Part model, mm, in its own coordinate system. A direction names the side the tool comes from. Round coordinates to 2 decimals unless told otherwise and drop trailing zeros. Loops run counter-clockwise (first coordinate to the right, second up) from the corner with the lowest first, then second, coordinate; pieces in that order, holes last.
Autodesk Inventor part; units mm, degrees
ref_plane "YZ Plane" through (0, 0, 0) normal (1, 0, 0) x (0, 1, 0)
ref_plane "XZ Plane" through (0, 0, 0) normal (0, 1, 0) x (-1, 0, 0)
ref_plane "XY Plane" through (0, 0, 0) normal (0, 0, 1) x (1, 0, 0)
sketch "Sketch1" plane through (0, 0, 0) normal (0, 1, 0) x (-1, 0, 0)
  line L0 (12.5, 12) -> (-12.5, 12)
  line L1 (-12.5, 12) -> (-12.5, -12)
  line L2 (-12.5, -12) -> (12.5, -12)
  line L3 (12.5, -12) -> (12.5, 12)
  line L4 (12.5, 12) -> (-12.5, -12) construction
  line L5 (-12.5, 12) -> (12.5, -12) construction
  point P0 (0, 0)
  dimension "d0" = 25
  dimension "d1" = 24
extrude "Extrusion1" add sketch "Sketch1" along normal blind 1
sketch "Sketch2" plane through (0, 1, 0) normal (0, 1, 0) x (1, 0, 0)
  line L0 (-12.5, 12) -> (-10.5, 12)
  line L1 (-10.5, 12) -> (-10.5, 10)
  line L2 (-10.5, 10) -> (-12.5, 10)
  line L3 (-12.5, 10) -> (-12.5, 12)
  line L4 (12.5, 12) -> (10.5, 12)
  line L5 (10.5, 12) -> (10.5, 10)
  line L6 (10.5, 10) -> (12.5, 10)
  line L7 (12.5, 10) -> (12.5, 12)
  line L8 (-12.5, 12) -> (-10.5, 12)
  line L9 (-10.5, 12) -> (-10.5, -2.5)
  line L10 (-10.5, -2.5) -> (-12.5, -2.5)
  line L11 (-12.5, -2.5) -> (-12.5, 12)
  line L12 (12.5, 12) -> (10.5, 12)
  line L13 (10.5, 12) -> (10.5, -2.5)
  line L14 (10.5, -2.5) -> (12.5, -2.5)
  line L15 (12.5, -2.5) -> (12.5, 12)
  circle A0 centre (-10.5, 10) radius 1
  circle A1 centre (-10.5, -2.5) radius 1
  circle A2 centre (10.5, -2.5) radius 1
  circle A3 centre (10.5, 10) radius 1
  point P0 (0, 0)
  dimension "d4" = 2
  dimension "d5" = 2
  dimension "d6" = 2
  dimension "d7" = 2
  dimension "d8" = 14.5
  dimension "d9" = 14.5
  dimension "d10" = 2
  dimension "d11" = 2
  dimension "d12" = 2
  dimension "d13" = 2
extrude "Extrusion2" cut sketch "Sketch2" against normal up to next contours A0 L9 L1 | L1 L2 A0 | L2 L9 A0 | A1 L9 L10 | L10 L9 A1 | A3 L6 L5 | L5 L13 A3 | A3 L13 L6 | A2 L13 L14 | L14 L13 A2
sketch "Sketch3" plane through (0, 1, 0) normal (0, 1, 0) x (1, 0, 0)
  circle A0 centre (-10.5, -2.5) radius 1
  circle A1 centre (10.5, -2.5) radius 1
  line L0 (-12.5, 12) -> (-12.5, -12)
  line L1 (-10.5, -2.5) -> (10.5, -2.5)
  line L2 (-4, -6.5) -> (4, -6.5)
  line L3 (4, -6.5) -> (4, 1.5)
  line L4 (4, 1.5) -> (-4, 1.5)
  line L5 (-4, 1.5) -> (-4, -6.5)
  line L6 (-4, -6.5) -> (4, 1.5) construction
  line L7 (4, -6.5) -> (-4, 1.5) construction
  point P0 (0, 0)
  point P1 (0, -2.5)
  dimension "d16" = 8
  dimension "d17" = 8
extrude "Extrusion3" add sketch "Sketch3" along normal blind 1 contours L5 L4 L3 L1 | L1 L3 L2 L5
sketch "Sketch4" plane through (0, 2, 0) normal (0, 1, 0) x (1, 0, 0)
  line L0 (-4, 1.5) -> (4, -6.5)
  circle A0 centre (0, -2.5) radius 3.5
  point P0 (0, 0)
  dimension "d20" = 7
extrude "Extrusion4" add sketch "Sketch4" along normal blind 4
sketch "Sketch5" plane through (0, 6, 2.5) normal (0, 1, 0) x (1, 0, 0)
  circle A0 centre (0, 0) radius 3.5
  circle A1 centre (0, 0) radius 2.5
  point P0 (0, 2.5)
  dimension "d23" = 5
extrude "Extrusion5" cut sketch "Sketch5" against normal blind 1 contours A1
properties part number "kamera"
1) Wall check: line 1 along X through (y, z) = (0.55, -10); line 2 along Z through (x, y) = (-10.5, 0.65); line 3 along Y through (x, z) = (2.25, 9.5). Give the ranges that are in metal, low to high.
Values:
line 1: x = -12.5 to -11.5, -9.5 to 9.5, 11.5 to 12.5
line 2: z = -12 to -11, -9 to 1.5, 3.5 to 12
line 3: y = 0 to 1
2) Slice it at D-D, the plane z = 2.5. Give the cut face in (x, y), then the cut area to 3 significant figures.
Values:
outline: (-12.5, 0) - (-11.5, 0) - (-11.5, 1) - (-12.5, 1) - close; (-9.5, 0) - (9.5, 0) - (9.5, 1) - (4, 1) - (4, 2) - (3.5, 2) - (3.5, 6) - (2.5, 6) - (2.5, 5) - (-2.5, 5) - (-2.5, 6) - (-3.5, 6) - (-3.5, 2) - (-4, 2) - (-4, 1) - (-9.5, 1) - close; (11.5, 0) - (12.5, 0) - (12.5, 1) - (11.5, 1) - close
area: 52.0 mm2
3) Slice it at B-B, the plane x = 10.5. Give the cut face in (y, z).
Values:
outline: (0, -12) - (1, -12) - (1, -11) - (0, -11) - close; (0, -9) - (1, -9) - (1, 1.5) - (0, 1.5) - close; (0, 3.5) - (1, 3.5) - (1, 12) - (0, 12) - close
4) Mould opens along X. For faces 4 (the face through (-10.63, 0.51, -10.99)), 5 (the face through (0.2, 0.5, -12)), 6 (the face through (12.5, 0.5, 0.2)), 7 (the face through (-2, 5.5, 4)) say: released by +X, released by -X, zero draft, split by the parting line, or undercut.
Values:
face 4: undercut
face 5: zero draft
face 6: released by +X
face 7: undercut
5) Slice it at C-C, the plane y = 0.65. Give the cut face in (x, z), then the cut area to 3 significant figures.
Values:
outline: (-12.5, -12) - (12.5, -12) - (12.5, 12) - (-12.5, 12) - close; hole circle Ø2 at (-10.5, -10); hole circle Ø2 at (-10.5, 2.5); hole circle Ø2 at (10.5, -10); hole circle Ø2 at (10.5, 2.5)
area: 587 mm2
6) Drop flat-ended pins along their axis: pin 1 Ø3 at (x, z) = (10.5, 2.5) entering from +Y; pin 2 Ø12 at (x, z) = (5.5, -6) entering from +Y; pin 3 Ø0.5 at (y, z) = (1.5, 4) entering from -X. Give the stop position or say it passes through.
Values:
pin 1: stops at y = 1
pin 2: stops at y = 2
pin 3: stops at x = -4
7) Slice it at A-A, the plane z = -10. Give the cut face in (x, y).
Values:
outline: (-12.5, 0) - (-11.5, 0) - (-11.5, 1) - (-12.5, 1) - close; (-9.5, 0) - (9.5, 0) - (9.5, 1) - (-9.5, 1) - close; (11.5, 0) - (12.5, 0) - (12.5, 1) - (11.5, 1) - close
8) Tool access for faces 1 (the face through (0.1, 1.5, -1.5)), 2 (the face through (0, 5, 2)), 3 (the face through (4, 1.5, 2.6)): list every direction of +Z, -Z, +X, -X, +Y, -Y with a clear straight run to the whole face (end or side of a thin tool).
Values:
face 1: -Z, +X, -X, +Y
face 2: +Y
face 3: +Z, -Z, +X, +Y
